from build123d import *

# Parameters (mm, degrees)
SKETCH1_R           = 11
BOSS_EXTRUDE1_DEPTH = 21.7
SKETCH7_R           = 12.25
BOSS_EXTRUDE6_DEPTH = 6
SKETCH8_R           = 15
BOSS_EXTRUDE7_DEPTH = 14.5
CUT_EXTRUDE4_DEPTH  = 21.7
BOSS_EXTRUDE8_DEPTH = 9.3


with BuildPart() as part:
    # Sketch1 → Boss-Extrude1 (new body)
    with BuildSketch(Plane(origin=(0, 0, 0), x_dir=(1, 0, 0), z_dir=(0, 1, 0))):
        with Locations(Location((0, 0, 0), (0, 0, 270))):
            Circle(SKETCH1_R)
    extrude(amount=BOSS_EXTRUDE1_DEPTH)

    # Sketch7 → Boss-Extrude6 (add)
    with BuildSketch(Plane(origin=(0, 21.7, 0), x_dir=(1, 0, 0), z_dir=(0, 1, 0))):
        with Locations(Location((0, 0, 0), (0, 0, 270))):
            Circle(SKETCH7_R)
    extrude(amount=BOSS_EXTRUDE6_DEPTH)

    # Sketch8 → Boss-Extrude7 (add)
    with BuildSketch(Plane(origin=(0, 27.7, 0), x_dir=(1, 0, 0), z_dir=(0, 1, 0))):
        with Locations(Location((0, 0, 0), (0, 0, 90))):
            Circle(SKETCH8_R)
    extrude(amount=BOSS_EXTRUDE7_DEPTH)

    # Sketch3 → Cut-Extrude4 (cut)
    with BuildSketch(Plane.XZ):
        with BuildLine():
            Line((-4.958555581, 9.818998246), (-10.469742362, 3.374091709))
            ThreePointArc((-10.469742362, 3.374091709), (-8.360161447, 7.148965), (-4.958555581, 9.818998246))
        make_face()
        with BuildLine():
            Line((10.469742362, -3.374091709), (4.958555581, -9.818998246))
            ThreePointArc((4.958555581, -9.818998246), (8.360161447, -7.148965), (10.469742362, -3.374091709))
        make_face()
    extrude(amount=-CUT_EXTRUDE4_DEPTH, mode=Mode.SUBTRACT)

    # Sketch9 → Boss-Extrude8 (add)
    with BuildSketch(Plane.XZ):
        Polygon((8.013326492, -2.707706192), (8.621338234, -3.227630919), (4.526931006, -8.015723384), (3.918919265, -7.495798657), align=None)
        Polygon((-3.918903937, 7.495816582), (-4.526915678, 8.015741309), (-8.621322906, 3.227648844), (-8.013311164, 2.707724116), align=None)
    extrude(amount=BOSS_EXTRUDE8_DEPTH)


solid = part.part
Part model, mm, in its own coordinate system. A direction names the side the tool comes from. Coordinates: 2 decimals unless noted, no trailing zeros. Order: outer loops, then holes, each group sorted by start corner. A loop starts at its lowest first (then second) coordinate and runs counter-clockwise, first axis right, second up.
(1) Slice it at B-B, the plane x = -0.75. Write the cut outline in (y, z), and give its area (3 significant figures).
Check sheet entries:
outline: (0, -10.97) - (21.7, -10.97) - (21.7, -12.23) - (27.7, -12.23) - (27.7, -14.98) - (42.2, -14.98) - (42.2, 14.98) - (27.7, 14.98) - (27.7, 12.23) - (21.7, 12.23) - (21.7, 10.97) - (0, 10.97) - close
area: 1,060 mm2
(2) Pin check, flat tips, straight feed: pin 1 Ø12 at (y, z) = (1.5, 10) entering from -X; pin 2 Ø2 at (x, y) = (4.5, 30) entering from -Z; pin 3 Ø6 at (x, y) = (-1.5, 14.5) entering from -Z. Stop position of each tip, or through.
Check sheet entries:
pin 1: stops at x = -9.93
pin 2: stops at z = -14.59
pin 3: stops at z = -11
(3) Probe L1, parallel to Y at x = -4, z = 1.75; L2, parallel to Y at x = 11.25, z = 3.5; L3, parallel to X at y = 30.5, z = -11.5. List the from-to ranges inside material, lowest first.
Check sheet entries:
L1: y = 0 to 42.2
L2: y = 21.7 to 42.2
L3: x = -9.63 to 9.63
(4) Slice it at C-C, the plane y = 38. Write the cut outline in (x, z), and give its area (3 significant figures).
Check sheet entries:
outline: circle Ø30 at (0, 0)
area: 707 mm2
(5) Tool access for faces 1 (the face through (11, 27.7, 6)), 2 (the face through (5.937, -4.585, -5.135)), 3 (the face through (7.753, 10.698, -6.551)): list every direction of +Z, -Z, +X, -X, +Y, -Y with a clear straight run to the whole face (end or side of a thin tool).
Check sheet entries:
face 1: -Y
face 2: +Z, -X, -Y
face 3: -Z, +X, -Y
(6) Slice it at D-D, the plane z = -6.25. Write the cut outline in (x, y).
Check sheet entries:
outline: (-13.64, 27.7) - (-10.54, 27.7) - (-10.54, 21.7) - (-9.05, 21.7) - (-9.05, 0) - (4.98, 0) - (4.98, -9.3) - (6.04, -9.3) - (6.04, 0) - (8.01, 0) - (8.01, 21.7) - (10.54, 21.7) - (10.54, 27.7) - (13.64, 27.7) - (13.64, 42.2) - (-13.64, 42.2) - close
(7) Slice it at A-A, the plane z = 0. Write the cut outline in (x, y).
Check sheet entries:
outline: (-15, 27.7) - (-12.25, 27.7) - (-12.25, 21.7) - (-11, 21.7) - (-11, 0) - (11, 0) - (11, 21.7) - (12.25, 21.7) - (12.25, 27.7) - (15, 27.7) - (15, 42.2) - (-15, 42.2) - close
